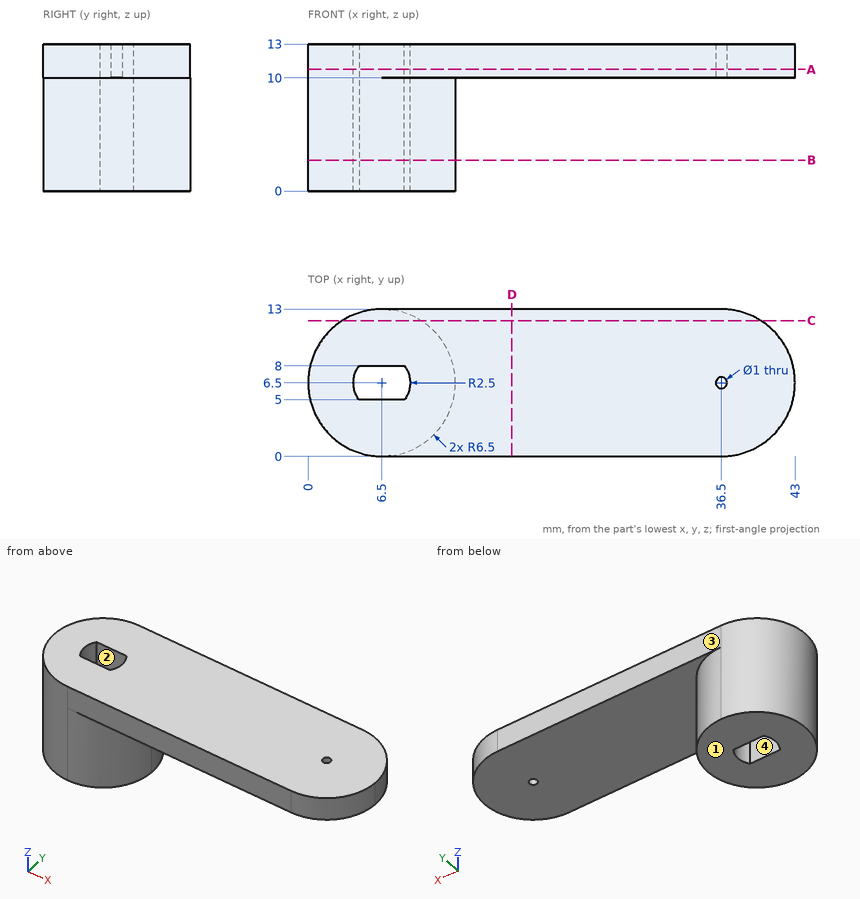
Here's the drawing with two shaded views (mm, measured from the low corner). I have some questions. A direction names the side the tool comes from. Give positions to 0.01 mm unless a question says otherwise; leave off trailing zeros. Order: outer loops, then holes, each group sorted by start corner. A loop starts at its lowest first (then second) coordinate and runs counter-clockwise, first axis right, second up. Notation, with made-up numbers: M -17,50.5 L 33,50.5 A20 cw 33,85.5 Z; hole C 64,72.5 d6. An arc over 180 degrees is marked long. Answer as a JSON object with one key per item and string values. Group by question number.
1) Suppose I cut it at D-D, the plane x = 18. Write out the boundary of the cut face in (y, z).
2) Please list where these lines run through material, in increasing order: L1, parallel to Y at x = 36.5, z = 10.8; L2, parallel to Z at x = 24, y = 7; L3, parallel to X at y = 6.5, z = 3.25. Write a range as [from, to].
3) We'd pull the mould along X, two halves only. Please class the marked faces 3 and 4: pulls with the +X half, pulls with the -X half, needs draft (parallel to the pull), parting line crosses it, or undercut.
4) On a 3-axis mill with a long thin cutter (end or side, diameter ignored), from which of +Z, -Z, +X, -X, +Y, -Y can I reach the whole of each face in a straight line? I mean the marked faces 1 and 2. Say none if no direction works.
5) Suppose I cut it at A-A, the plane z = 10.75. Write out the boundary of the cut face in (x, y), plus the area to 3 significant figures.
6) I'm going to push flat-ended pins straight in: pin 1 Ø1 at (y, z) = (10, 10) entering from -X; pin 2 Ø3 at (x, z) = (13, 7.5) entering from -Y. Where does each tip first touch, or does it pass through?
7) Suppose I cut it at C-C, the plane y = 12. Write out the boundary of the cut face in (x, z).
8) Suppose I cut it at B-B, the plane z = 2.75. Write out the boundary of the cut face in (x, y), plus the area to 3 significant figures.
Results found:
{
 "1": {"outline": "M 0,10 L 13,10 L 13,13 L 0,13 Z"},
 "2": {"L1": "[0, 6], [7, 13]", "L2": "[10, 13]", "L3": "[0, 4], [9, 13]"},
 "3": {"face 3": "needs draft", "face 4": "undercut"},
 "4": {"face 1": "-Z, +X, -X, +Y, -Y", "face 2": "+Z, -Z"},
 "5": {"outline": "M 6.5,0 L 36.5,0 A6.5 ccw 36.5,13 L 6.5,13 A6.5 ccw Z; hole M 4.5,5 L 8.5,5 A2.5 ccw 8.5,8 L 4.5,8 A2.5 ccw Z; hole C 36.5,6.5 d1", "area": "508 mm²"},
 "6": {"pin 1": "x = 0.73", "pin 2": "y = 2.35"},
 "7": {"outline": "M 3.04,0 L 9.96,0 L 9.96,10 L 39.96,10 L 39.96,13 L 3.04,13 Z"},
 "8": {"outline": "C 6.5,6.5 d13; hole M 4.5,5 L 8.5,5 A2.5 ccw 8.5,8 L 4.5,8 A2.5 ccw Z", "area": "119 mm²"}
}
